Geometry check sheet. Reference: drawing and pictorial views, mm from the part's lowest x, y, z. A direction names the side the tool comes from. Round coordinates to 2 decimals unless told otherwise and drop trailing zeros. Loops run counter-clockwise (first coordinate to the right, second up) from the corner with the lowest first, then second, coordinate; pieces in that order, holes last. Notation, with made-up numbers: M -20.75,20 L -16.75,20 A20 ccw -16.75,34 Z; hole C 70,24 d1. An arc over 180 degrees is marked long. One line per question, with ' | ' between items. Start each with the question number.
(1) Section check C-C (x = 23). Record the boundary of the cut face in (y, z).
(2) Go/stop test with flat-tipped pins: P1, Ø3, axis at x = 41.5, y = 4, coming from the +Z side; P2, Ø2.5, axis at x = 8.97, z = 9.32, coming from the +Y side; P3, Ø1, axis at y = 4.5, z = 30, coming from the -X side; P4, Ø2, axis at y = 3.5, z = 5, coming from the -X side. Record where each tip stops, or that it passes through.
(3) Tool access check on the marked faces 4 and 5. Record the directions out of +Z, -Z, +X, -X, +Y, -Y that give a thin tool (end or side, any length) a straight path to the whole face; none if there is none.
(4) Section check A-A (z = 14.5). Count the separate pieces of the cut face and the enclosed holes in it, and give its area (3 significant figures).
(5) Draft check along Z on the marked faces 1, 2 and 3. Enter one of: +Z half, -Z half, draft (parallel to the pull), parting line (faces both ways), or undercut.
(6) Thickness scan on probe 1 along X at (y, z) = (1.5, 17.5) (1 decimal); probe 2 along X at (y, z) = (5, 13) (1 decimal); probe 3 along X at (y, z) = (4, 30.5) (1 decimal). Record the ranges inside material, lowest first. Write a range as [from, to].
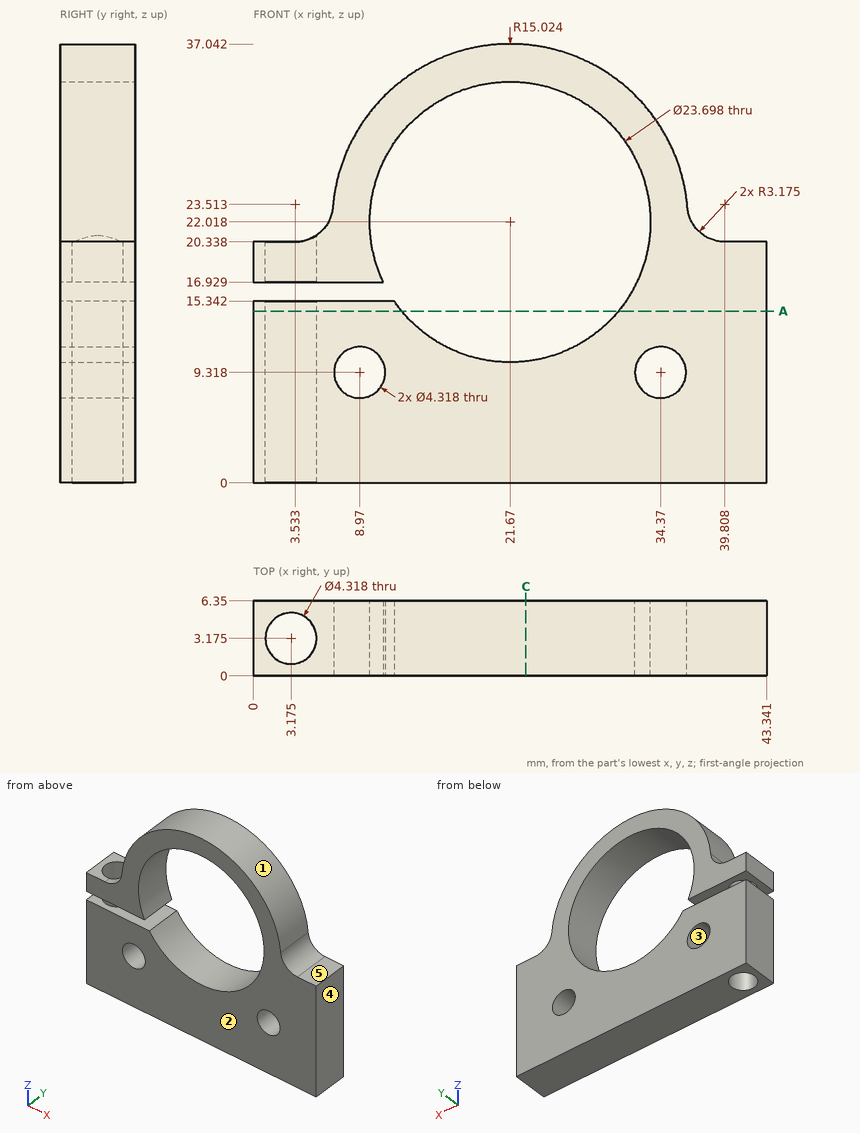
The answers:
1) outline: M 0,0 L 6.35,0 L 6.35,10.24 L 0,10.24 Z; M 0,33.79 L 6.35,33.79 L 6.35,36.98 L 0,36.98 Z
2) P1: z = 20.34 | P2: through | P3: x = 8.64 | P4: x = 0
3) face 4: +Z, -Z, +X, +Y, -Y | face 5: +Z, +X, +Y, -Y
4) separate pieces: 2 | enclosed holes: 1 | area: 144 mm²
5) face 1: +Z half | face 2: draft | face 3: undercut
6) probe 1: [0, 1.8], [4.5, 10.7], [32.6, 43.3] | probe 2: [0, 2], [4.3, 14], [29.4, 43.3] | probe 3: [9.3, 13.4], [29.9, 34.1]
